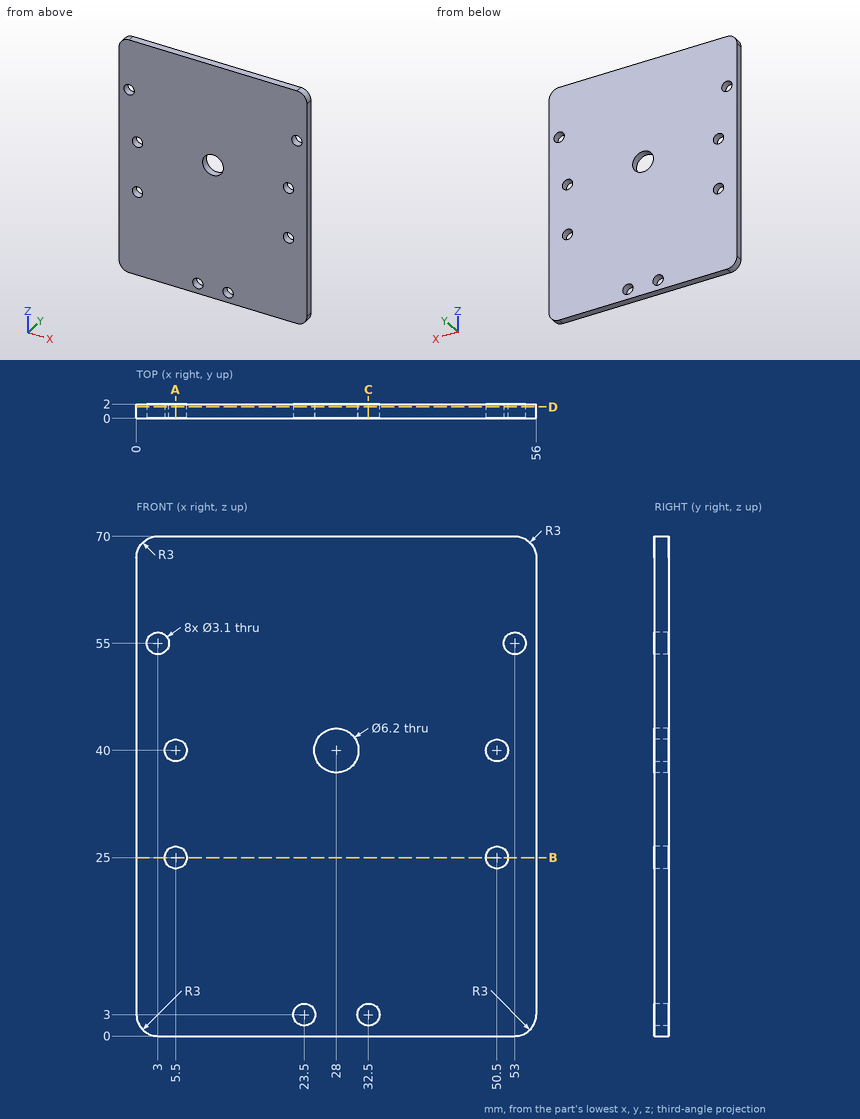
Part print with two shaded views. Sizes in mm from the minimum x, y, z corner. Round coordinates to 2 decimals unless told otherwise and drop trailing zeros. Order: outer loops, then holes, each group sorted by start corner. A loop starts at its lowest first (then second) coordinate and runs counter-clockwise, first axis right, second up. Notation, with made-up numbers: (25.5, 25) - (30.5, 25) arc R25 ccw to (30.5, 38) - close; hole circle Ø11 at (37, -16.75). An arc over 180 degrees is marked (long way). Answer as CSV lines item,"result". Start each with the question number.
1. Saw through at B-B, the plane z = 25. Write the cut outline in (x, y).
2. Drill centre lines: L1, parallel to X at y = 1.2, z = 25; L2, parallel to Z at x = 50.5, y = 0.6; L3, parallel to X at y = 1.5, z = 3. Where is each one in solid material? Low to high. Write a range as [from, to].
3. Saw through at A-A, the plane x = 5.5. Write the cut outline in (y, z), and give its area (3 significant figures).
4. Saw through at D-D, the plane y = 1.6. Count the separate pieces of the cut face and the enclosed holes in it, and give its area (3 significant figures).
5. Saw through at C-C, the plane x = 32.5. Write the cut outline in (y, z), and give its area (3 significant figures).
Model answer:
1,outline,"(0, 0) - (3.95, 0) - (3.95, 2) - (0, 2) - close; (7.05, 0) - (48.95, 0) - (48.95, 2) - (7.05, 2) - close; (52.05, 0) - (56, 0) - (56, 2) - (52.05, 2) - close"
2,L1,"x = [0, 3.95], [7.05, 48.95], [52.05, 56]"
2,L2,"z = [0, 23.45], [26.55, 38.45], [41.55, 70]"
2,L3,"x = [0, 21.95], [25.05, 30.95], [34.05, 56]"
3,outline,"(0, 0) - (2, 0) - (2, 23.45) - (0, 23.45) - close; (0, 26.55) - (2, 26.55) - (2, 38.45) - (0, 38.45) - close; (0, 41.55) - (2, 41.55) - (2, 70) - (0, 70) - close"
3,area,"128 mm²"
4,separate pieces,"1"
4,enclosed holes,"9"
4,area,"3,820 mm²"
5,outline,"(0, 0) - (2, 0) - (2, 1.45) - (0, 1.45) - close; (0, 4.55) - (2, 4.55) - (2, 70) - (0, 70) - close"
5,area,"134 mm²"
